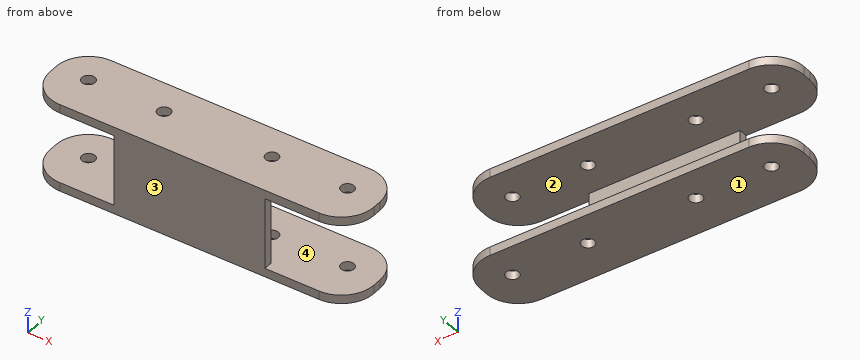
```python
from build123d import *

# Parameters (mm, degrees)
EXTRUDE_1_DEPTH     = 150
SKETCH_2_R          = 3
CUT_EXTRUDE_1_DEPTH = 300
SKETCH_3_W          = 40
SKETCH_3_H          = 33
CUT_EXTRUDE_2_DEPTH = 10
FILLET_1_R          = 15
SKETCH_4_R          = 3
CUT_EXTRUDE_3_DEPTH = 160.176003217


with BuildPart() as part:
    # 草图1 → 凸台-拉伸1 (new body)
    with BuildSketch(Plane(origin=(0, 0, 0), x_dir=(0, 0, -1), z_dir=(1, 0, 0))):
        Polygon((-16.5, 4), (-16.5, 34), (-20.5, 34), (-20.5, 0), (0, 0), (0, 4), align=None)
        Polygon((16.5, 4), (0, 4), (0, 0), (20.5, 0), (20.5, 34), (16.5, 34), align=None)
    extrude(amount=EXTRUDE_1_DEPTH)

    # 草图2 → 切除-拉伸1 (cut)
    with BuildSketch(Plane.XY.offset(20.5)):
        with Locations(Location((15, 19, 0), (0, 0, 90))):
            Circle(SKETCH_2_R)
        with Locations(Location((135, 19, 0), (0, 0, 90))):
            Circle(SKETCH_2_R)
    extrude(amount=-CUT_EXTRUDE_1_DEPTH, mode=Mode.SUBTRACT)

    # 草图3 → 切除-拉伸2 (cut)
    with BuildSketch(Plane.XZ):
        with Locations((130, 0)):
            Rectangle(SKETCH_3_W, SKETCH_3_H)
        with Locations((20, 0)):
            Rectangle(SKETCH_3_W, SKETCH_3_H)
    extrude(amount=-CUT_EXTRUDE_2_DEPTH, mode=Mode.SUBTRACT)

    # 圆角1
    fillet_1_edges = [part.edges().sort_by_distance(p)[0] for p in [
        (0, 0, 18.5),
        (0, 34, 18.5),
        (150, 34, 18.5),
        (150, 0, 18.5),
        (150, 34, -18.5),
        (150, 0, -18.5),
        (0, 0, -18.5),
        (0, 34, -18.5),
    ]]
    fillet(fillet_1_edges, radius=FILLET_1_R)

    # 草图4 → 切除-拉伸3 (cut, through all)
    with BuildSketch(Plane.XY.offset(20.5)):
        with Locations((50, 19)):
            Circle(SKETCH_4_R)
        with Locations((100, 19)):
            Circle(SKETCH_4_R)
    extrude(amount=-CUT_EXTRUDE_3_DEPTH, mode=Mode.SUBTRACT)


solid = part.part
```
Read the model definition and answer for the solid it produces. Units are mm, in the model's axes. Face numbers are marked on the shaded views. Coordinates: 2 decimals unless noted, no trailing zeros. Write each loop counter-clockwise with the first axis right and the second up, starting at its lowest first coordinate (ties: lowest second). Pieces come first, ordered by that corner, then holes. Notation, with made-up numbers: (-15.75, 12) -> (42.25, 12) arc R20 cw to (42.25, 23) -> close; hole circle Ø2 at (2, 43.5). An arc over 180 degrees is marked (long way). Write item = value, one per line.
(1) Given pin 1 Ø1 at (x, z) = (25.5, 15) entering from +Y; pin 2 Ø4.5 at (y, z) = (2, 0.5) entering from -X; pin 3 Ø10 at (x, z) = (87.5, -8) entering from +Y; pin 4 Ø3 at (y, z) = (2, -4.5) entering from +X, each flat-ended and moving along its own axis, determine where each tip first touches the part or whether it passes through.
From the geometry:
pin_1 = through
pin_2 = 40
pin_3 = 4
pin_4 = 110
(2) For a pull along Z with two mould halves and no side action, classify the marked faces 1, 2, 3 and 4 as +Z half, -Z half, draft (parallel to the pull), parting line (faces both ways), or undercut.
From the geometry:
face_1 = -Z half
face_2 = undercut
face_3 = draft
face_4 = undercut
(3) Straight lines are drawn through the part: L1, parallel to Z at x = 127.5, y = 6.5; L2, parallel to Y at x = 135, z = -19.4; L3, parallel to Y at x = 86.5, z = 0. For each, find the intervals that lie inside material, in ascending order. Write a range as from..to.
From the geometry:
L1 = -20.5..-16.5, 16.5..20.5
L2 = 0..16, 22..34
L3 = 0..4
(4) Section A-A on x = 100 is taken. Write down the section's boundary in (y, z).
From the geometry:
outline = (0, -20.5) -> (16, -20.5) -> (16, -16.5) -> (4, -16.5) -> (4, 16.5) -> (16, 16.5) -> (16, 20.5) -> (0, 20.5) -> close; (22, -20.5) -> (34, -20.5) -> (34, -16.5) -> (22, -16.5) -> close; (22, 16.5) -> (34, 16.5) -> (34, 20.5) -> (22, 20.5) -> close
(5) Section D-D on x = 62 is taken. Write down the section's boundary in (y, z), plus the area to 3 significant figures.
From the geometry:
outline = (0, -20.5) -> (34, -20.5) -> (34, -16.5) -> (4, -16.5) -> (4, 16.5) -> (34, 16.5) -> (34, 20.5) -> (0, 20.5) -> close
area = 404 mm2
(6) Section B-B on y = 10 is taken. Write down the section's boundary in (x, z).
From the geometry:
outline = (0.86, -20.5) -> (149.14, -20.5) -> (149.14, -16.5) -> (0.86, -16.5) -> close; (0.86, 16.5) -> (149.14, 16.5) -> (149.14, 20.5) -> (0.86, 20.5) -> close
(7) Section C-C on x = 141 is taken. Write down the section's boundary in (y, z).
From the geometry:
outline = (1.25, -20.5) -> (32.75, -20.5) -> (32.75, -16.5) -> (1.25, -16.5) -> close; (1.25, 16.5) -> (32.75, 16.5) -> (32.75, 20.5) -> (1.25, 20.5) -> close
